Read the model definition and answer for the solid it produces. Units are mm, in the model's axes. Face numbers are marked on the shaded views. Coordinates: 2 decimals unless noted, no trailing zeros. Loops run counter-clockwise (first coordinate to the right, second up) from the corner with the lowest first, then second, coordinate; pieces in that order, holes last. Notation, with made-up numbers: (69.25, 79.5) - (107.25, 79.5) arc R34 ccw to (107.25, 116.5) - close; hole circle Ø1 at (49.25, 60.5). An arc over 180 degrees is marked (long way). Use one line per item in the form item = value. Start each with the question number.
1) The mould has two halves that part along X. Classify the marked faces 1, 2 and 3: released by +X, released by -X, zero draft, split by the parting line, or undercut.
2) A cutting plane is placed at C-C (x = -26). Give the vertices of the cut face in (y, z), and give its area (3 significant figures).
3) Each of these flat-tipped pins is pushed along its axis until it touches: P1, Ø4, axis at y = -19.5, z = 5.5, coming from the -X side; P2, Ø10, axis at x = -76, y = -2.5, coming from the -Z side. Where does it stop, or does it pass through?
4) A cutting plane is placed at A-A (z = 3.25). Give the vertices of the cut face in (x, y), and give its area (3 significant figures).
5) A cutting plane is placed at B-B (x = -140.5). Give the vertices of the cut face in (y, z).
6) Consider line 1 (Y direction, x = -134.5, z = 6.5); line 2 (Y direction, x = -122, z = 3.5); line 3 (X direction, y = -14.75, z = 6.5). Determine where each line is inside the solid, lowest interval first.
from build123d import *

# Parameters (mm, degrees)
BOSS_EXTRUDE1_DEPTH = 6.8


with BuildPart() as part:
    # Sketch1 → Boss-Extrude1 (new body)
    with BuildSketch(Plane.XY):
        with BuildLine():
            Line((-3.736553352, -0.105475371), (0, 0))
            Line((0, 0), (0.260408581, -9.22519204))
            ThreePointArc((0.260408581, -9.22519204), (-1.360098109, -14.970948565), (-5.965617029, -18.769495059))
            ThreePointArc((-5.965617029, -18.769495059), (-20.103980037, -23.096122462), (-34.787070991, -24.833894972))
            Line((-34.787070991, -24.833894972), (-46.296555972, -25.15878454))
            Line((-46.296555972, -25.15878454), (-46.909976525, -22.174905175))
            Line((-46.909976525, -22.174905175), (-55.197899778, -22.408856547))
            Line((-55.197899778, -22.408856547), (-55.292212243, -19.06775851))
            ThreePointArc((-55.292212243, -19.06775851), (-57.168585337, -14.876394082), (-61.459123685, -13.239448011))
            Line((-61.459123685, -13.239448011), (-86.952751483, -13.959081751))
            ThreePointArc((-86.952751483, -13.959081751), (-119.784800915, -12.909412184), (-152.397282866, -8.976055209))
            ThreePointArc((-152.397282866, -8.976055209), (-156.666477303, -6.118238551), (-157.834820075, -1.115428104))
            Line((-157.834820075, -1.115428104), (-157.390699994, 1.898303501))
            Line((-157.390699994, 1.898303501), (-153.450231486, 2.009534988))
            Line((-153.450231486, 2.009534988), (-152.767576007, -1.311125833))
            Line((-152.767576007, -1.311125833), (-122.028102345, -0.443412436))
            ThreePointArc((-122.028102345, -0.443412436), (-100.521194384, -1.324753836), (-79.098250735, 0.768410766))
            Line((-79.098250735, 0.768410766), (-55.870655521, 1.424078972))
            ThreePointArc((-55.870655521, 1.424078972), (-34.68336237, -0.227804683), (-13.432310629, -0.379167061))
            Line((-13.432310629, -0.379167061), (-11.903069428, -4.205729222))
            Line((-11.903069428, -4.205729222), (-4.406055716, -3.994103632))
            Line((-4.406055716, -3.994103632), (-3.736553352, -0.105475371))
        make_face()
    extrude(amount=BOSS_EXTRUDE1_DEPTH)


solid = part.part
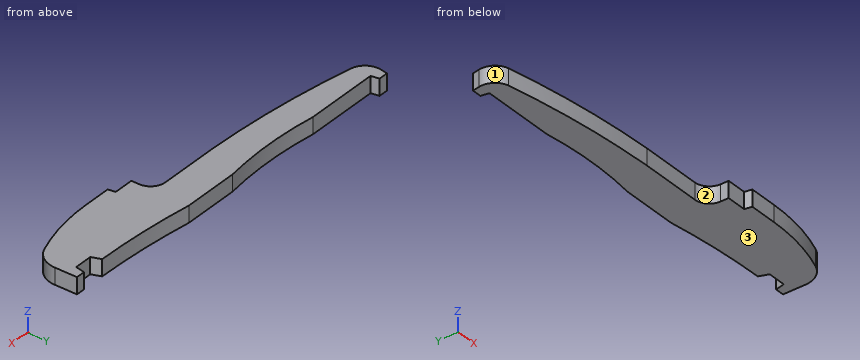
Found:
q1.face_1 = released by -X
q1.face_2 = undercut
q1.face_3 = zero draft
q2.outline = (-24.12, 0) - (-0.47, 0) - (-0.47, 6.8) - (-24.12, 6.8) - close
q2.area = 161 mm^2
q3.P1 = -55.55
q3.P2 = 0
q4.outline = (-157.83, -1.12) arc R7 ccw to (-152.4, -8.98) arc R373.11 ccw to (-86.95, -13.96) - (-61.46, -13.24) arc R6 cw to (-55.29, -19.07) - (-55.2, -22.41) - (-46.91, -22.17) - (-46.3, -25.16) - (-34.79, -24.83) arc R82.63 ccw to (-5.97, -18.77) arc R10 ccw to (0.26, -9.23) - (0, 0) - (-3.74, -0.11) - (-4.41, -3.99) - (-11.9, -4.21) - (-13.43, -0.38) arc R300.71 cw to (-55.87, 1.42) - (-79.1, 0.77) arc R155.7 cw to (-122.03, -0.44) - (-152.77, -1.31) - (-153.45, 2.01) - (-157.39, 1.9) - close
q4.area = 2,470 mm^2
q5.outline = (-10.75, 0) - (-0.96, 0) - (-0.96, 6.8) - (-10.75, 6.8) - close
q6.line_1 = -11.5 to -0.8
q6.line_2 = -12.73 to -0.45
q6.line_3 = -57.31 to -1.22
